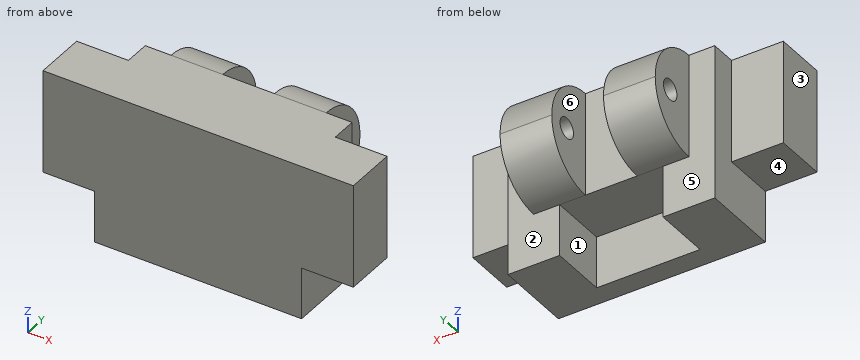
from build123d import *

# Parameters (mm, degrees)
F0_W     = 100
F0_H     = 12.5
F1_DEPTH = 50
F2_W     = 25
F2_H     = 50
F3_DEPTH = 25
F4_R     = 24.99999
F5_R     = 5
F6_DEPTH = 112.501
F7_W     = 50
F7_H     = 10
F8_DEPTH = 75


# Not quite as in the source:
# - a fillet or chamfer is up to 0.001 mm smaller than in the source, because OpenCascade refuses the exact size


with BuildPart() as f1:
    # F0 (on Top) → F1 (new body)
    with BuildSketch(Plane.XY):
        Polygon((75, -12.5), (75, 12.5), (50, 12.5), (50, 0), (-50, 0), (-50, 12.5), (-75, 12.5), (-75, -12.5), align=None)
        with Locations((0, 6.25)):
            Rectangle(F0_W, F0_H)
        with Locations((0, 18.75)):
            Rectangle(F0_W, F0_H)
    extrude(amount=F1_DEPTH)

    # F2 (on face) → F3 (join)
    with BuildSketch(Plane(origin=(0, 25, 0), x_dir=(-1, 0, 0), z_dir=(0, 1, 0))):
        with Locations((-25, 25)):
            Rectangle(F2_W, F2_H)
        with Locations((25, 25)):
            Rectangle(F2_W, F2_H)
    extrude(amount=F3_DEPTH)

    # F4 (radius 25 in the source; OpenCascade refuses exactly that, so slightly less here)
    f4_edges = [f1.edges().sort_by_distance(p)[0] for p in [
        (25, 50, 50),
        (25, 50, 0),
        (-25, 50, 0),
        (-25, 50, 50),
    ]]
    fillet(f4_edges, radius=F4_R)

    # F5 (on face) → F6 (cut, through all)
    with BuildSketch(Plane.YZ.offset(37.5)):
        with Locations((38.875002414, 25)):
            Circle(F5_R)
    extrude(amount=-F6_DEPTH, mode=Mode.SUBTRACT)

    # F7 (on face) → F8 (join)
    with BuildSketch(Plane.XY.offset(50)):
        Polygon((25, 25), (25, -2.5), (25, -12.5), (50, -12.5), (50, 12.5), (50, 25), (37.5, 25), align=None)
        with Locations((0, -7.5)):
            Rectangle(F7_W, F7_H)
        Polygon((-37.5, 25), (-50, 25), (-50, 12.5), (-50, -12.5), (-25, -12.5), (-25, -2.5), (-25, 25), align=None)
    extrude(amount=-F8_DEPTH)


solid = f1.part
Verification items for the finished model (mm, model axes). Face numbers are marked on the shaded views. A direction names the side the tool comes from. Coordinates: 2 decimals unless noted, no trailing zeros. Loops run counter-clockwise (first coordinate to the right, second up) from the corner with the lowest first, then second, coordinate; pieces in that order, holes last. Notation, with made-up numbers: M 83.5,3 L 141.5,3 A23 cw 141.5,15 Z; hole C -17.5,-13.75 d6. An arc over 180 degrees is marked long. One line per item, written item: value.
1. Section check D-D on y = 26.5. Record the cut outline in (x, z).
Answers follow:
outline: M -37.5,0.05 L -12.5,0.05 L -12.5,49.95 L -37.5,49.95 Z; M 12.5,0.05 L 37.5,0.05 L 37.5,49.95 L 12.5,49.95 Z
2. Section check C-C on z = -13. Record the cut outline in (x, y).
Answers follow:
outline: M -50,-12.5 L 50,-12.5 L 50,25 L 25,25 L 25,-2.5 L -25,-2.5 L -25,25 L -50,25 Z
3. Material ranges on line 1 along X through (y, z) = (35, 37); line 2 along Y through (x, z) = (-6.5, 27); line 3 along X through (y, z) = (-5.5, -16), recorded low to high. Write a range as from..to.
Answers follow:
line 1: -37.5..-12.5, 12.5..37.5
line 2: -12.5..25
line 3: -50..50
4. Mould release check, pull along X, two halves, no side actions. Record for the marked faces 1, 2 and 3: pulls with the +X half, pulls with the -X half, needs draft (parallel to the pull), parting line crosses it, or undercut.
Answers follow:
face 1: undercut
face 2: needs draft
face 3: pulls with the -X half
5. Gauge pin test, flat ends, axial feed: P1, Ø6, axis at y = 30.5, z = 26, coming from the -X side; P2, Ø6, axis at x = -12, y = 37.5, coming from the +Z side; P3, Ø16, axis at y = 38.88, z = 25, coming from the +X side. Record the tip position at first contact, or that the pin passes through.
Answers follow:
P1: x = -37.5
P2: z = 48.11
P3: x = 37.5
6. Section check B-B on y = 7. Record the cut outline in (x, z).
Answers follow:
outline: M -75,0 L -50,0 L -50,-25 L -25,-25 L -25,0 L 25,0 L 25,-25 L 50,-25 L 50,0 L 75,0 L 75,50 L -75,50 Z
7. Set-up check for the marked faces 4, 5 and 6: record each of +Z, -Z, +X, -X, +Y, -Y from which the full face is reachable in a straight line by a thin tool's end or side.
Answers follow:
face 4: -Z, -X, +Y, -Y
face 5: -Z, -X, +Y
face 6: +Z, -Z, +Y
